from build123d import *

# Parameters (mm, degrees)
SKETCH_1_R          = 50
EXTRUDE_1_DEPTH     = 50
SKETCH_2_R          = 44
CUT_EXTRUDE_1_DEPTH = 36.5
CUT_EXTRUDE_START   = -9.5
SKETCH_3_R          = 44
CUT_EXTRUDE_2_DEPTH = 9.5
SKETCH_4_R          = 14.75
SKETCH_4_R_2        = 1.5
CUT_EXTRUDE_3_DEPTH = 4
CUT_EXTRUDE_4_DEPTH = 4
FILLET_1_R          = 5


with BuildPart() as part:
    # 草图1 → 凸台-拉伸1 (new body)
    with BuildSketch(Plane(origin=(0, 0, 0), x_dir=(1, 0, 0), z_dir=(0, 1, 0))):
        with Locations(Location((0, 0, 0), (0, 0, 270))):
            Circle(SKETCH_1_R)
    extrude(amount=EXTRUDE_1_DEPTH)

    # 草图2 → 切除-拉伸1 (cut)
    with BuildSketch(Plane(origin=(0, 50, 0), x_dir=(1, 0, 0), z_dir=(0, 1, 0))):
        with Locations(Location((0, 0, 0), (0, 0, 270))):
            Circle(SKETCH_2_R)
    extrude(amount=-CUT_EXTRUDE_1_DEPTH, mode=Mode.SUBTRACT)

    # 草图3 → 切除-拉伸2 (cut)
    with BuildSketch(Plane.XZ.offset(CUT_EXTRUDE_START)):
        with Locations(Location((0, 0, 0), (0, 0, 90))):
            Circle(SKETCH_3_R)
    extrude(amount=CUT_EXTRUDE_2_DEPTH, mode=Mode.SUBTRACT)

    # 草图4 → 切除-拉伸3 (cut)
    with BuildSketch(Plane(origin=(0, 13.5, 0), x_dir=(1, 0, 0), z_dir=(0, 1, 0))):
        with Locations(Location((0, 0, 0), (0, 0, 270))):
            Circle(SKETCH_4_R)
        with Locations(Location((0, 17.5, 0), (0, 0, 270))):
            Circle(SKETCH_4_R_2)
        with Locations(Location((12.374368671, 12.374368671, 0), (0, 0, 270))):
            Circle(SKETCH_4_R_2)
        with Locations(Location((17.5, 0, 0), (0, 0, 270))):
            Circle(SKETCH_4_R_2)
        with Locations(Location((12.374368671, -12.374368671, 0), (0, 0, 270))):
            Circle(SKETCH_4_R_2)
        with Locations(Location((0, -17.5, 0), (0, 0, 270))):
            Circle(SKETCH_4_R_2)
        with Locations(Location((-12.374368671, -12.374368671, 0), (0, 0, 270))):
            Circle(SKETCH_4_R_2)
        with Locations(Location((-17.5, 0, 0), (0, 0, 270))):
            Circle(SKETCH_4_R_2)
        with Locations(Location((-12.374368671, 12.374368671, 0), (0, 0, 270))):
            Circle(SKETCH_4_R_2)
    extrude(amount=-CUT_EXTRUDE_3_DEPTH, mode=Mode.SUBTRACT)

    # 草图8 → 切除-拉伸4 (cut)
    with BuildSketch(Plane(origin=(0, 13.5, 0), x_dir=(1, 0, 0), z_dir=(0, 1, 0))):
        with BuildLine():
            Line((-11.25, 19.485571585), (-20, 34.641016151))
            ThreePointArc((-20, 34.641016151), (0, 40), (20, 34.641016151))
            Line((20, 34.641016151), (11.25, 19.485571585))
            ThreePointArc((11.25, 19.485571585), (0, 22.5), (-11.25, 19.485571585))
        make_face()
        with BuildLine():
            Line((19.485571585, 11.25), (34.641016151, 20))
            ThreePointArc((34.641016151, 20), (40, 0), (34.641016151, -20))
            Line((34.641016151, -20), (19.485571585, -11.25))
            ThreePointArc((19.485571585, -11.25), (22.5, 0), (19.485571585, 11.25))
        make_face()
        with BuildLine():
            Line((11.25, -19.485571585), (20, -34.641016151))
            ThreePointArc((20, -34.641016151), (0, -40), (-20, -34.641016151))
            Line((-20, -34.641016151), (-11.25, -19.485571585))
            ThreePointArc((-11.25, -19.485571585), (0, -22.5), (11.25, -19.485571585))
        make_face()
        with BuildLine():
            Line((-19.485571585, -11.25), (-34.641016151, -20))
            ThreePointArc((-34.641016151, -20), (-40, 0), (-34.641016151, 20))
            Line((-34.641016151, 20), (-19.485571585, 11.25))
            ThreePointArc((-19.485571585, 11.25), (-22.5, 0), (-19.485571585, -11.25))
        make_face()
    extrude(amount=-CUT_EXTRUDE_4_DEPTH, mode=Mode.SUBTRACT)

    # 圆角1
    fillet_1_edges = [part.edges().sort_by_distance(p)[0] for p in [
        (-11.25, 11.5, 19.485571585),
        (11.25, 11.5, 19.485571585),
        (20, 11.5, 34.641016151),
        (-20, 11.5, 34.641016151),
        (19.485571585, 11.5, 11.25),
        (19.485571585, 11.5, -11.25),
        (34.641016151, 11.5, -20),
        (34.641016151, 11.5, 20),
        (-19.485571585, 11.5, -11.25),
        (-19.485571585, 11.5, 11.25),
        (-34.641016151, 11.5, 20),
        (-34.641016151, 11.5, -20),
        (11.25, 11.5, -19.485571585),
        (-11.25, 11.5, -19.485571585),
        (-20, 11.5, -34.641016151),
        (20, 11.5, -34.641016151),
    ]]
    fillet(fillet_1_edges, radius=FILLET_1_R)


solid = part.part
Verification items for the finished model (mm, model axes). Give positions to 0.01 mm unless a question says otherwise; leave off trailing zeros. Write each loop counter-clockwise with the first axis right and the second up, starting at its lowest first coordinate (ties: lowest second). Pieces come first, ordered by that corner, then holes. Notation, with made-up numbers: M 13,81.25 L 19,81.25 A21 ccw 19,109.25 Z; hole C -39.75,37 d8. An arc over 180 degrees is marked long. Put each result on its own line as item: value. Start each with the question number.
1. Section check C-C (y = 34). Record the cut outline in (x, z).
2. Go/stop test with flat-tipped pins: pin 1 Ø6 at (x, y) = (12.5, 27.5) entering from +Z; pin 2 Ø12 at (x, z) = (-3.5, -21) entering from +Y; pin 3 Ø8 at (y, z) = (11, 19) entering from -X. Record where each tip stops, or that it passes through.
3. Draft check along Z on faces 1 (the face through (15.02, 24.65, 47.69)), 2 (the face through (-44.2, 0, -0.2)), 3 (the face through (-1, 9.5, 19)). Enter one of: +Z half, -Z half, draft (parallel to the pull), parting line (faces both ways), or undercut.
4. Scan lines: line 1 along X through (y, z) = (11, 0); line 2 along Z through (x, y) = (17, 10); line 3 along Y through (x, z) = (25, 29). Record each from-to range of solid material in increasing order. Write a range as [from, to].
5. Section check A-A (x = 0). Give the number of separate pieces and of enclosed holes in the cut face, and give its area (3 significant figures).
6. Section check D-D (z = -27). Record the cut outline in (x, y), and give its area (3 significant figures).
Answer list:
1. outline: C 0,0 d100; hole C 0,0 d88
2. pin 1: z = 49.09
2. pin 2: y = 13.5
2. pin 3: x = -47.7
3. face 1: parting line
3. face 2: draft
3. face 3: undercut
4. line 1: [-50, -40], [-22.5, -19], [-16, -14.75], [14.75, 16], [19, 22.5], [40, 50]
4. line 2: [-47.02, -35.49], [-29.44, -1.41], [1.41, 29.44], [35.49, 47.02]
4. line 3: [9.5, 13.5]
5. separate pieces: 6
5. enclosed holes: 0
5. area: 670 mm2
6. outline: M -42.08,0 L -34.74,0 L -34.74,9.5 L -15.59,9.5 L -15.59,13.5 L -34.74,13.5 L -34.74,50 L -42.08,50 Z; M 15.59,9.5 L 34.74,9.5 L 34.74,0 L 42.08,0 L 42.08,50 L 34.74,50 L 34.74,13.5 L 15.59,13.5 Z
6. area: 887 mm2
